Read the model definition and answer for the solid it produces. Units are mm, in the model's axes. Face numbers are marked on the shaded views. A direction names the side the tool comes from. Coordinates: 2 decimals unless noted, no trailing zeros. Write each loop counter-clockwise with the first axis right and the second up, starting at its lowest first coordinate (ties: lowest second). Pieces come first, ordered by that corner, then holes. Notation, with made-up numbers: (61, -25) -> (103, -25) arc R24 cw to (103, 5) -> close; hole circle Ø2 at (-22, 84.5). An arc over 180 degrees is marked (long way). Write item = value, one per line. Start each with the question number.
1) A tool of negligible diameter and unlimited length cuts with its end or side. For the marked faces 1 and 2, from which of +Z, -Z, +X, -X, +Y, -Y can it reach the whole face along a straight path? Write none if from no direction.
2) Section A-A (x = -67.5) is taken. Determine the outline of the cut face in (y, z), plus the area to 3 significant figures.
3) For a pull along Z with two mould halves and no side action, classify the marked faces 3, 4, 5 and 6 as released by +Z, released by -Z, zero draft, split by the parting line, or undercut.
4) Find the intervals of material crossed by line 1 along Z through (x, y) = (-67.5, 12.5); line 2 along Y through (x, z) = (-61.75, -5.5); line 3 along Z through (x, y) = (-67.25, 14.75), in increasing order. Write a range as from..to.
5) Section C-C (z = 5.75) is taken. Determine the outline of the cut face in (x, y), plus the area to 3 significant figures.
6) Section D-D (y = 19.5) is taken. Determine the outline of the cut face in (x, z).
7) Flat-ended cylindrical pins translate along their axes: pin 1 Ø3.5 at (y, z) = (13, 0) entering from +X; pin 2 Ø8 at (y, z) = (14, 0) entering from +X. Find the tip coordinate at first contact, or state that the pin passes through.
8) Section B-B (y = 10.75) is taken. Determine the outline of the cut face in (x, z), plus the area to 3 significant figures.
from build123d import *

# Parameters (mm, degrees)
BOSS_EXTRUDE1_DEPTH = 25
SKETCH2_R           = 3
CUT_EXTRUDE1_DEPTH  = 25
SKETCH3_W           = 25
SKETCH3_H           = 25
BOSS_EXTRUDE2_DEPTH = 5


with BuildPart() as part:
    # Sketch1 → Boss-Extrude1 (new body)
    with BuildSketch(Plane(origin=(0, 0, 0), x_dir=(1, 0, 0), z_dir=(0, 1, 0))):
        with BuildLine():
            Line((-65.504745346, 11.478381524), (-65.504745346, -13.521618476))
            Line((-65.504745346, -13.521618476), (-70.504745346, -13.521618476))
            ThreePointArc((-70.504745346, -13.521618476), (-71.536999603, -1.021618476), (-70.504745346, 11.478381524))
            Line((-70.504745346, 11.478381524), (-65.504745346, 11.478381524))
        make_face()
    extrude(amount=BOSS_EXTRUDE1_DEPTH)

    # Sketch2 → Cut-Extrude1 (cut)
    with BuildSketch(Plane(origin=(-65.504745346, 0, 0), x_dir=(0, 0, -1), z_dir=(1, 0, 0))):
        with Locations((-1.021618476, 12.5)):
            Circle(SKETCH2_R)
    extrude(amount=-CUT_EXTRUDE1_DEPTH, mode=Mode.SUBTRACT)

    # Sketch3 → Boss-Extrude2 (add)
    with BuildSketch(Plane(origin=(-65.504745346, 0, 0), x_dir=(0, 0, -1), z_dir=(1, 0, 0))):
        with Locations((-1.021618476, 12.5)):
            Rectangle(SKETCH3_W, SKETCH3_H)
        Polygon((5.906584755, 12.5), (2.442483139, 18.5), (-4.485720091, 18.5), (-7.949821706, 12.5), (-4.485720091, 6.5), (2.442483139, 6.5), align=None, mode=Mode.SUBTRACT)
    extrude(amount=BOSS_EXTRUDE2_DEPTH)


solid = part.part
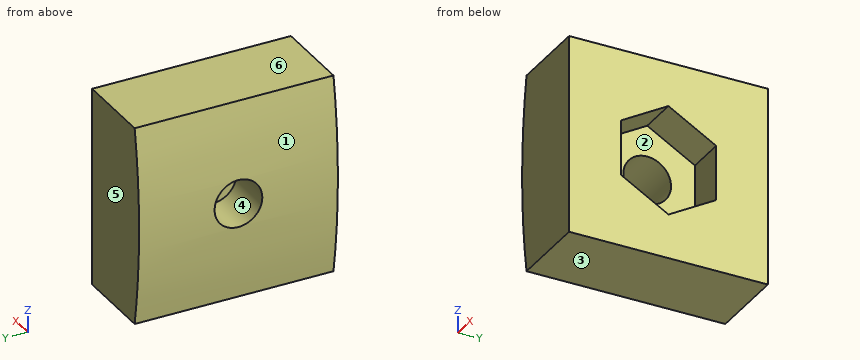
Answer key:
q1.face_1 = -X, +Y, -Y
q1.face_2 = +X
q2.outline = (0, -11.48) -> (25, -11.48) -> (25, 13.52) -> (0, 13.52) -> close; hole circle Ø6 at (12.5, 1.02)
q2.area = 597 mm^2
q3.face_3 = released by -Z
q3.face_4 = undercut
q3.face_5 = zero draft
q3.face_6 = released by +Z
q4.line_1 = -11.48..-1.98, 4.02..13.52
q4.line_2 = 0..11.8, 13.2..25
q4.line_3 = -11.48..-0.96, 3.01..13.52
q5.outline = (-71.39, 0) -> (-60.5, 0) -> (-60.5, 8.69) -> (-65.5, 8.69) -> (-65.5, 16.31) -> (-60.5, 16.31) -> (-60.5, 25) -> (-71.39, 25) -> close
q5.area = 234 mm^2
q6.outline = (-70.5, -11.48) -> (-60.5, -11.48) -> (-60.5, 13.52) -> (-70.5, 13.52) arc R76.2 ccw to start
q7.pin_1 = through
q7.pin_2 = -65.5
q8.outline = (-71.5, -1.42) arc R76.2 ccw to (-70.5, -11.48) -> (-60.5, -11.48) -> (-60.5, -4.9) -> (-65.5, -4.9) -> (-65.5, -1.42) -> close; (-71.5, 3.46) -> (-65.5, 3.46) -> (-65.5, 6.94) -> (-60.5, 6.94) -> (-60.5, 13.52) -> (-70.5, 13.52) arc R76.2 ccw to start
q8.area = 179 mm^2
